from build123d import *

# Parameters (mm, degrees)
SKETCH3_R           = 37.5
SKETCH3_R_2         = 30.5
BOSS_EXTRUDE1_DEPTH = 192
CUT_EXTRUDE3_START  = -41
SKETCH7_R           = 39
SKETCH7_R_2         = 34
CUT_EXTRUDE3_DEPTH  = 110


with BuildPart() as part:
    # Sketch3 → Boss-Extrude1 (new body)
    with BuildSketch(Plane(origin=(0, 0, 0), x_dir=(1, 0, 0), z_dir=(0, 1, 0))):
        Circle(SKETCH3_R)
        Circle(SKETCH3_R_2, mode=Mode.SUBTRACT)
    extrude(amount=BOSS_EXTRUDE1_DEPTH)

    # Sketch7 → Cut-Extrude3 (cut)
    with BuildSketch(Plane(origin=(0, 0, 0), x_dir=(-1, 0, 0), z_dir=(0, -1, 0)).offset(CUT_EXTRUDE3_START)):
        Circle(SKETCH7_R)
        Circle(SKETCH7_R_2, mode=Mode.SUBTRACT)
    extrude(amount=-CUT_EXTRUDE3_DEPTH, mode=Mode.SUBTRACT)


solid = part.part
Source: CAD feature listing. Evaluate the final solid. Frame: model axes, mm. A direction names the side the tool comes from. Coordinates: 2 decimals unless noted, no trailing zeros. Loops run counter-clockwise (first coordinate to the right, second up) from the corner with the lowest first, then second, coordinate; pieces in that order, holes last. Notation, with made-up numbers: (49.5, 88.25) - (92.5, 88.25) arc R13 cw to (92.5, 108.25) - close; hole circle Ø2 at (30.5, 55.5). An arc over 180 degrees is marked (long way). One line per item, written item: value. Start each with the question number.
1. Contact query for flat-ended pins moving along their axis: P1, Ø1, axis at x = 13.5, y = 56, coming from the +Z side; P2, Ø1.5, axis at x = 25.5, z = 13.5, coming from the -Y side; P3, Ø5, axis at y = 143, z = 29, coming from the +X side; P4, Ø10, axis at y = 114.5, z = 13, coming from the +X side. Output: stop coordinate, or through.
2. Set-up query: faces 5 (the cylindrical face through (-18.28, 95.23, -28.67)), 6 (the cylindrical face through (-4.88, 20.21, -37.18)). Return all of +Z, -Z, +X, -X, +Y, -Y with unobstructed straight access to the full face (end or side cutting, diameter ignored); none if empty.
3. Ray query, L1, parallel to Y at x = -30.5, z = -20.5; L2, parallel to X at y = 150, z = 0. Return the intervals inside material, ascending.
4. Section A-A (z = 0). Return the cut outline in (x, y).
5. Section C-C (y = 104). Return the cut outline in (x, z).
6. Mould query, pull axis Y, two halves, no side actions, for faces 1 (the flat face through (5.4, 192, 30.4)), 2 (the cylindrical face through (-24.204, 94.656, 18.559)), 3 (the flat face through (-8.2, 41, 33.2)), 4 (the flat face through (5.4, 0, 30.4)). Classes: pulls with the +Y half, pulls with the -Y half, needs draft (parallel to the pull), parting line crosses it, or undercut.
7. Section B-B (x = 0). Return the cut outline in (y, z).
8. Section D-D (y = 156). Return the cut outline in (x, z), and give its area (3 significant figures).
Verdict:
1. P1: stops at z = 31.42
1. P2: passes through
1. P3: stops at x = 21.3
1. P4: stops at x = 33.05
2. face 5: none
2. face 6: +Y, -Y
3. L1: y = 0 to 41, 151 to 192
3. L2: x = -34 to -30.5, 30.5 to 34
4. outline: (-37.5, 0) - (-30.5, 0) - (-30.5, 192) - (-37.5, 192) - (-37.5, 151) - (-34, 151) - (-34, 41) - (-37.5, 41) - close; (30.5, 0) - (37.5, 0) - (37.5, 41) - (34, 41) - (34, 151) - (37.5, 151) - (37.5, 192) - (30.5, 192) - close
5. outline: circle Ø68 at (0, 0); hole circle Ø61 at (0, 0)
6. face 1: pulls with the +Y half
6. face 2: needs draft
6. face 3: undercut
6. face 4: pulls with the -Y half
7. outline: (0, -37.5) - (41, -37.5) - (41, -34) - (151, -34) - (151, -37.5) - (192, -37.5) - (192, -30.5) - (0, -30.5) - close; (0, 30.5) - (192, 30.5) - (192, 37.5) - (151, 37.5) - (151, 34) - (41, 34) - (41, 37.5) - (0, 37.5) - close
8. outline: circle Ø75 at (0, 0); hole circle Ø61 at (0, 0)
8. area: 1,500 mm2
